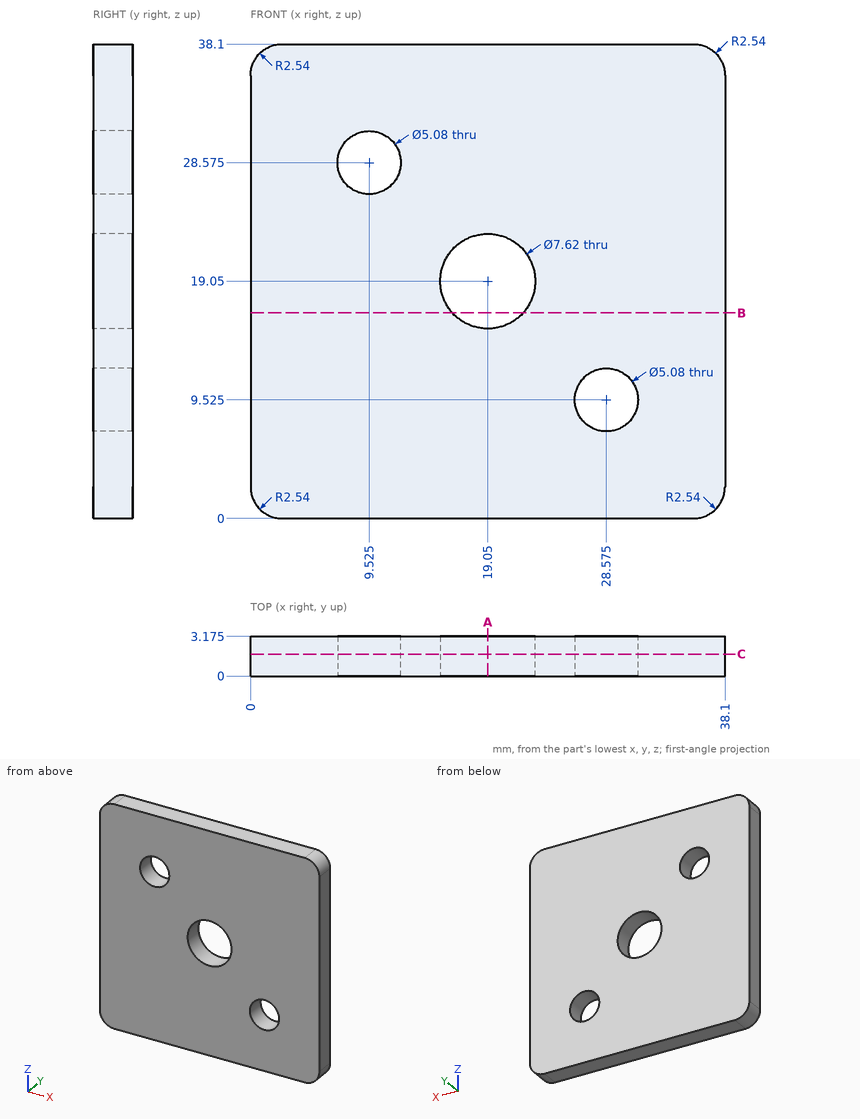
Job drawing, mm, ordinate dimensions from the low corner. One solid piece. Coordinates: 2 decimals unless noted, no trailing zeros. Write each loop counter-clockwise with the first axis right and the second up, starting at its lowest first coordinate (ties: lowest second). Pieces come first, ordered by that corner, then holes.
Item 1: Slice it at B-B (z = 16.5). Write the cut outline in (x, y) (3 decimals).
Item 2: Pin check, flat tips, straight feed: pin 1 (8 mm diameter, centred on x = 28.575, z = 9.525, fed in from -Y); pin 2 (7 mm diameter, centred on x = 19.05, z = 19.05, fed in from +Y) (1 decimal). Stop position of each tip, or through.
Item 3: Slice it at C-C (y = 1.75). Write the cut outline in (x, z) (3 decimals), and give its area (3 significant figures).
Item 4: Probe line 1 (Z direction, x = 19.05, y = 2.45); line 2 (Z direction, x = 16, y = 2.15). List the from-to ranges inside material, lowest first.
Item 5: Slice it at A-A (x = 19.05). Write the cut outline in (y, z) (3 decimals), and give its area (3 significant figures).
Results found:
1. outline: (0, 0) - (16.219, 0) - (16.219, 3.175) - (0, 3.175) - close; (21.881, 0) - (38.1, 0) - (38.1, 3.175) - (21.881, 3.175) - close
2. pin 1: stops at y = 0
2. pin 2: passes through
3. outline: (0, 2.54) arc R2.54 ccw to (2.54, 0) - (35.56, 0) arc R2.54 ccw to (38.1, 2.54) - (38.1, 35.56) arc R2.54 ccw to (35.56, 38.1) - (2.54, 38.1) arc R2.54 ccw to (0, 35.56) - close; hole circle Ø5.08 at (9.525, 28.575); hole circle Ø7.62 at (19.05, 19.05); hole circle Ø5.08 at (28.575, 9.525)
3. area: 1,360 mm2
4. line 1: z = 0 to 15.24, 22.86 to 38.1
4. line 2: z = 0 to 16.77, 21.33 to 38.1
5. outline: (0, 0) - (3.175, 0) - (3.175, 15.24) - (0, 15.24) - close; (0, 22.86) - (3.175, 22.86) - (3.175, 38.1) - (0, 38.1) - close
5. area: 96.8 mm2
